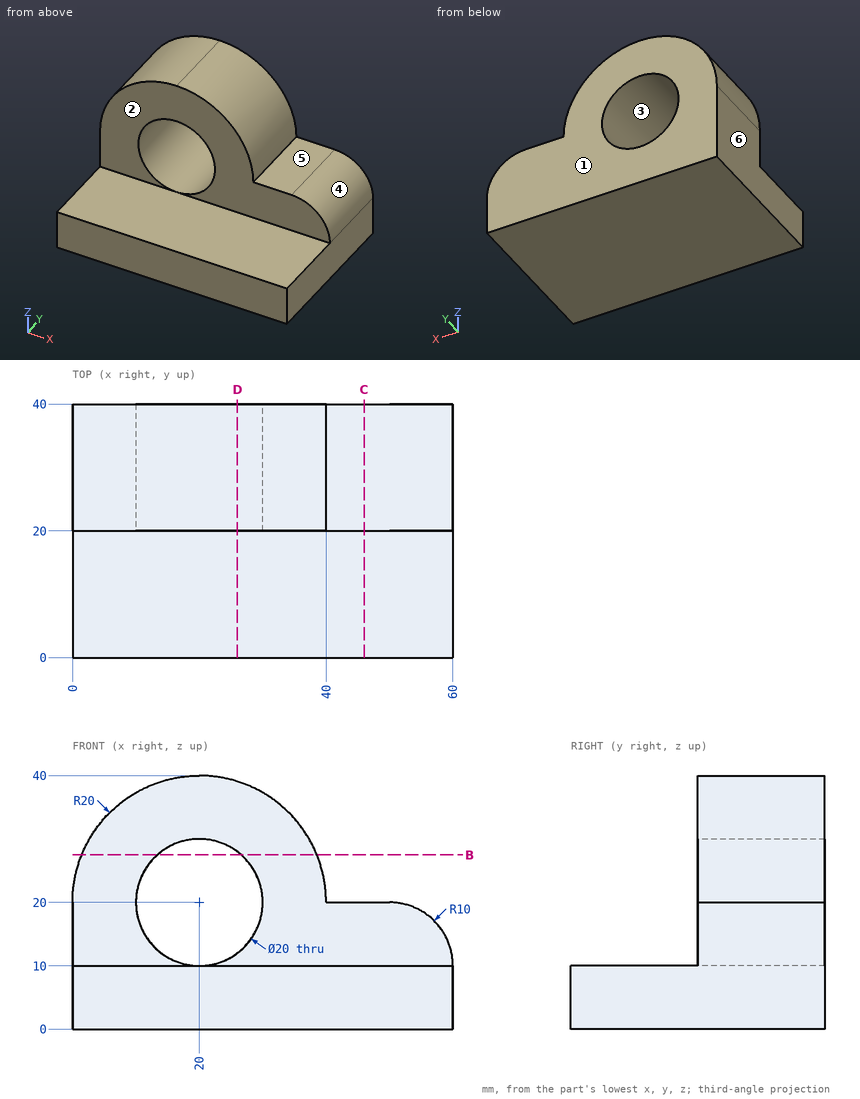
Study the drawing (mm; zero at the part's minimum x, y, z) and answer. A direction names the side the tool comes from. Give positions to 0.01 mm unless a question says otherwise; leave off trailing zeros. Loops run counter-clockwise (first coordinate to the right, second up) from the corner with the lowest first, then second, coordinate; pieces in that order, holes last. Notation, with made-up numbers: (-28.5, 63) -> (-10.5, 63) arc R20 ccw to (-10.5, 87) -> close; hole circle Ø5 at (60, -4). An arc over 180 degrees is marked (long way). Use a Markdown table: item, result. Add a question column.
1) The part is cut by section D-D, the plane x = 26. Determine the outline of the cut face in (y, z).
2) For a pull along X with two mould halves and no side action, classify the marked faces 3, 4, 5 and 6 as +X half, -X half, draft (parallel to the pull), parting line (faces both ways), or undercut.
3) Consider line 1 along Z through (x, y) = (20, 36); line 2 along Y through (x, z) = (29.5, 28); line 3 along Z through (x, y) = (37, 16.5). Determine where each line is inside the solid, lowest interval first.
4) Each of these flat-tipped pins is pushed along its axis until it touches: P1, Ø3, axis at x = 47, y = 30, coming from the +Z side; P2, Ø6, axis at x = 41.5, z = 23.5, coming from the -Y side; P3, Ø2, axis at y = 33, z = 33, coming from the -X side. Where does it stop, or does it pass through?
5) The part is cut by section C-C, the plane x = 46. Determine the outline of the cut face in (y, z), plus the area to 3 significant figures.
6) The part is cut by section B-B, the plane z = 27.5. Determine the outline of the cut face in (x, y), plus the area to 3 significant figures.
7) Which of the six approach directions +Z, -Z, +X, -X, +Y, -Y give full straight-line access (tool end or side, diameter ignored) to the marked faces 1 and 2?
Reported:
| question | item | result |
|---|---|---|
| 1 | outline | (0, 0) -> (40, 0) -> (40, 12) -> (20, 12) -> (20, 10) -> (0, 10) -> close; (20, 28) -> (40, 28) -> (40, 39.08) -> (20, 39.08) -> close |
| 2 | face 3 | undercut |
| 2 | face 4 | +X half |
| 2 | face 5 | draft |
| 2 | face 6 | -X half |
| 3 | line 1 | z = 0 to 10, 30 to 40 |
| 3 | line 2 | y = 20 to 40 |
| 3 | line 3 | z = 0 to 10 |
| 4 | P1 | stops at z = 20 |
| 4 | P2 | stops at y = 20 |
| 4 | P3 | stops at x = 4 |
| 5 | outline | (0, 0) -> (40, 0) -> (40, 20) -> (20, 20) -> (20, 10) -> (0, 10) -> close |
| 5 | area | 600 mm^2 |
| 6 | outline | (1.46, 20) -> (13.39, 20) -> (13.39, 40) -> (1.46, 40) -> close; (26.61, 20) -> (38.54, 20) -> (38.54, 40) -> (26.61, 40) -> close |
| 6 | area | 477 mm^2 |
| 7 | face 1 | +Z, -Z, +X, -X, +Y |
| 7 | face 2 | +Z, +X, -X, -Y |
